```python
from build123d import *

# Parameters (mm, degrees)
FILLET_1_R = 1.3


with BuildPart() as part:
    # Эскиз1 → Повернуть1 (revolve)
    with BuildSketch(Plane.XY):
        Polygon((-0.8, 1), (0.8, 1), (0.8, 3.25), (2.5, 3.25), (2.5, 0), (-2.5, 0), (-2.5, 3.25), (-0.8, 3.25), align=None)
    revolve(axis=Axis((0, -2, 0), (-1, 0, 0)))

    # Скругление1
    fillet_1_edges = [part.edges().sort_by_distance(p)[0] for p in [
        (2.5, -7.25, 0),
        (-2.5, -7.25, 0),
    ]]
    fillet(fillet_1_edges, radius=FILLET_1_R)


solid = part.part
```
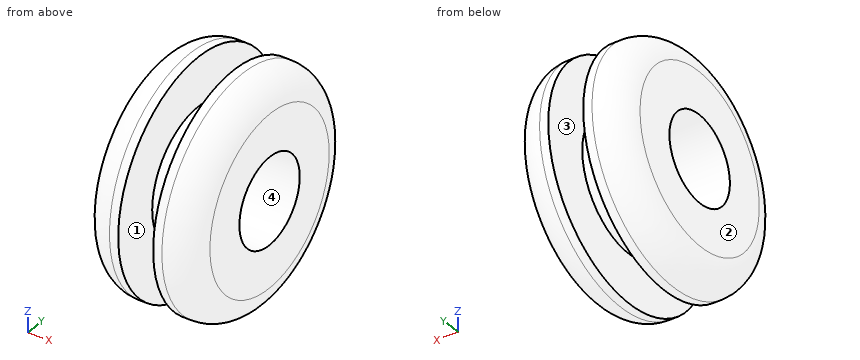
Build history of the part. All positions in model axes, mm. Face numbers are marked on the shaded views. A direction names the side the tool comes from. Coordinates: 2 decimals unless noted, no trailing zeros. Order: outer loops, then holes, each group sorted by start corner. A loop starts at its lowest first (then second) coordinate and runs counter-clockwise, first axis right, second up.
Item 1: Tool access for the marked faces 1 and 2: list every direction of +Z, -Z, +X, -X, +Y, -Y with a clear straight run to the whole face (end or side of a thin tool).
Filled in:
face 1: none
face 2: +Z, -Z, -X, +Y, -Y
Item 2: Mould opens along Y. For the marked faces 3 and 4 say: released by +Y, released by -Y, zero draft, split by the parting line, or undercut.
Filled in:
face 3: zero draft
face 4: undercut
Item 3: Saw through at C-C on x = 0.3. List the corners of the cut face in (y, z), then the cut area to 3 significant figures.
Filled in:
outline: circle Ø6 at (-2, 0); hole circle Ø4 at (-2, 0)
area: 15.7 mm2
Item 4: Drill centre lines: L1, parallel to Z at x = 0.6, y = -2; L2, parallel to X at y = 1.25, z = -0.5; L3, parallel to Y at x = -0.15, z = 0. Where is each one in solid material? Low to high.
Filled in:
L1: z = -3 to -2, 2 to 3
L2: x = -2.5 to -0.8, 0.8 to 2.5
L3: y = -5 to -4, 0 to 1
Item 5: Saw through at B-B on y = -2. List the corners of the cut face in (x, z), then the cut area to 3 significant figures.
Filled in:
outline: (-2.5, -3.95) arc R1.3 ccw to (-1.2, -5.25) - (-0.8, -5.25) - (-0.8, -3) - (0.8, -3) - (0.8, -5.25) - (1.2, -5.25) arc R1.3 ccw to (2.5, -3.95) - (2.5, -2) - (-2.5, -2) - close; (-2.5, 2) - (2.5, 2) - (2.5, 3.95) arc R1.3 ccw to (1.2, 5.25) - (0.8, 5.25) - (0.8, 3) - (-0.8, 3) - (-0.8, 5.25) - (-1.2, 5.25) arc R1.3 ccw to (-2.5, 3.95) - close
area: 23.8 mm2
Item 6: Saw through at D-D on x = -1.65. List the corners of the cut face in (y, z).
Filled in:
outline: circle Ø10.34 at (-2, 0); hole circle Ø4 at (-2, 0)
Item 7: Saw through at A-A on z = 0. List the corners of the cut face in (x, y).
Filled in:
outline: (-2.5, -5.95) arc R1.3 ccw to (-1.2, -7.25) - (-0.8, -7.25) - (-0.8, -5) - (0.8, -5) - (0.8, -7.25) - (1.2, -7.25) arc R1.3 ccw to (2.5, -5.95) - (2.5, -4) - (-2.5, -4) - close; (-2.5, 0) - (2.5, 0) - (2.5, 1.95) arc R1.3 ccw to (1.2, 3.25) - (0.8, 3.25) - (0.8, 1) - (-0.8, 1) - (-0.8, 3.25) - (-1.2, 3.25) arc R1.3 ccw to (-2.5, 1.95) - close
Item 8: Drop flat-ended pins along their axis: pin 1 Ø1 at (x, y) = (1.5, -1) entering from +Z; pin 2 Ø1.5 at (x, z) = (-1.5, -4) entering from -Y; pin 3 Ø3 at (x, y) = (-1, 1) entering from +Z. Give the stop position or say it passes through.
Filled in:
pin 1: stops at z = 5.22
pin 2: stops at y = -6.1
pin 3: stops at z = 5.03
